Input: part model. Units: mm. Frame: model coordinates. A direction names the side the tool comes from. Coordinates: 2 decimals unless noted, no trailing zeros. Loops run counter-clockwise (first coordinate to the right, second up) from the corner with the lowest first, then second, coordinate; pieces in that order, holes last.
(1) Set-up query: faces 4 (the face through (11.3, -6.096, -3.7)), 5 (the face through (8, 0, -11)), 6 (the face through (-9, 6.35, -7)), 7 (the face through (-4.18, 14.79, 10.09)), 8 (the face through (-13.239, 3.131, 6.886)). Return all of +Z, -Z, +X, -X, +Y, -Y with unobstructed straight access to the full face (end or side cutting, diameter ignored); none if empty.
(2) Contact query for flat-ended pins moving along their axis: P1, Ø12, axis at x = -7, y = 12.5, coming from the +Z side; P2, Ø3, axis at y = 5.5, z = -9, coming from the -X side; P3, Ø4, axis at y = 11, z = 4, coming from the +X side. Output: stop coordinate, or through.
(3) Mould query, pull axis X, two halves, no side actions, for faces 1 (the face through (-11, 14.605, -3)), 2 (the face through (0, -2.921, 0)), 3 (the face through (-13.937, 12.029, -3.095)). Classes: released by +X, released by -X, zero draft, split by the parting line, or undercut.
(4) Line query: L1, parallel to Y at x = -1, z = 10.25; L2, parallel to Z at x = 1.25, y = -4.75; L3, parallel to Y at x = -4.75, z = 13.5. Output: solid intervals per line, ascending.
(5) Section C-C, the plane y = 2. Return loops of the section in (x, z) (1 decimal), then the cut area to 3 significant figures.
(6) Section D-D, the plane y = -3.5. Return loops of the section in (x, z), then the cut area to 3 significant figures.
```python
from build123d import *

# Parameters (mm, degrees)
SKETCH1_R      = 14.9225
EXTRUDE1_DEPTH = 6.35
SKETCH3_R      = 11.049
EXTRUDE2_DEPTH = 9.271
SKETCH5_R      = 10.922
EXTRUDE3_DEPTH = 8.636
SKETCH6_R      = 14.27627633
EXTRUDE4_DEPTH = 5.08
SKETCH7_R      = 13.395629592
SKETCH7_R_2    = 11.049
EXTRUDE5_DEPTH = 6.096
EXTRUDE5_DRAFT = 6


with BuildPart() as part:
    # Sketch1 → Extrude1 (new body)
    with BuildSketch(Plane(origin=(0, 0, 0), x_dir=(1, 0, 0), z_dir=(0, 1, 0))):
        with Locations(Location((0, 0, 0), (0, 0, 270))):
            Circle(SKETCH1_R)
    extrude(amount=EXTRUDE1_DEPTH)

    # Sketch3 → Extrude2 (add)
    with BuildSketch(Plane(origin=(0, -2.921, 0), x_dir=(0, 0, -1), z_dir=(0, 1, 0))):
        with Locations(Location((0, 0, 0), (0, 0, 180))):
            Circle(SKETCH3_R)
    extrude(amount=EXTRUDE2_DEPTH)

    # Sketch4 → Revolve1 (revolve)
    with BuildSketch(Plane(origin=(0, 0, 0), x_dir=(0, 0, 1), z_dir=(1, 0, 0)), mode=Mode.PRIVATE) as revolve1_sk:
        Polygon((-11.049, 2.921), (-14.336865125, -1.171616093), (-11.049, -1.171616093), align=None)
    revolve(revolve1_sk.sketch.rotate(Axis((0, 1.376246897, 0), (0, -1, 0)), 180), axis=Axis((0, 1.376246897, 0), (0, -1, 0)))

    # Sketch5 → Extrude3 (add)
    with BuildSketch(Plane(origin=(0, 6.35, 0), x_dir=(-1, 0, 0), z_dir=(0, 1, 0))):
        with Locations(Location((0, 0, 0), (0, 0, 90))):
            Circle(SKETCH5_R)
    extrude(amount=EXTRUDE3_DEPTH)

    # Sketch6 → Extrude4 (add)
    with BuildSketch(Plane.ZX.offset(9.525)):
        Circle(SKETCH6_R)
    extrude(amount=EXTRUDE4_DEPTH)


with BuildPart() as extrude5_tool:
    # Sketch7 → Extrude5 (with draft: the straight prism first)
    with BuildSketch(Plane.XZ):
        Circle(SKETCH7_R)
        Circle(SKETCH7_R_2, mode=Mode.SUBTRACT)
    extrude(amount=EXTRUDE5_DEPTH)
    # Extrude5: the draft: its side faces are tilted about the plane it starts from
    extrude5_sides = [extrude5_tool.faces().sort_by_distance(p)[0] for p in [
        (-13.395629592, -3.048, 0),
        (-11.049, -3.048, 0),
    ]]
    draft(extrude5_sides, Plane.XZ, EXTRUDE5_DRAFT)


with BuildPart() as part_1:
    add(part.part)

    # Extrude5: add extrude5_tool
    add(extrude5_tool.part)


solid = part_1.part
```
Report:
1. face 4: +Z, -Z, +X, -X, -Y
1. face 5: -Y
1. face 6: none
1. face 7: +Y
1. face 8: +Y, -Y
2. P1: stops at z = 14.24
2. P2: stops at x = -12.9
2. P3: stops at x = 14.14
3. face 1: zero draft
3. face 2: undercut
3. face 3: split by the parting line
4. L1: y = -2.92 to 14.99
4. L2: z = -12.84 to -11.48, 11.48 to 12.84
4. L3: y = 0 to 6.35
5. outline: circle Ø29.8 at (0, 0)
5. area: 700 mm2
6. outline: circle Ø26.06 at (0, 0); hole circle Ø22.83 at (0, 0)
6. area: 124 mm2
